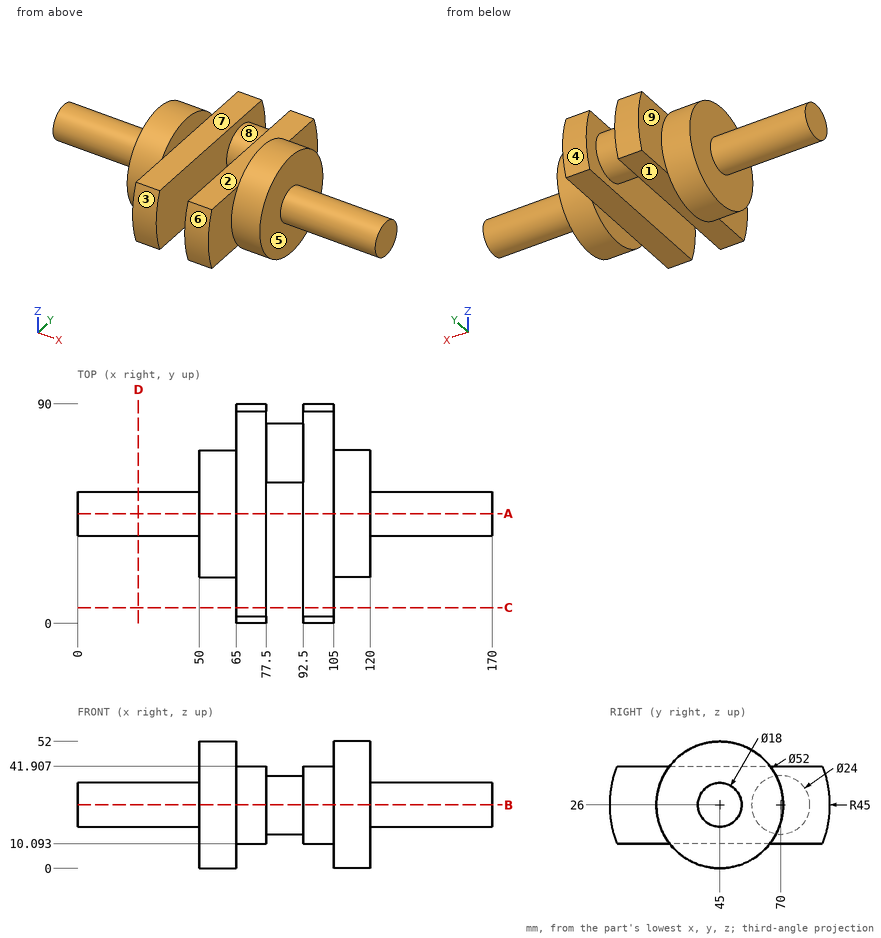
Check sheet for the drawn part. Datum: minimum x, y, z corner. Units: mm. A direction names the side the tool comes from. Give positions to 0.01 mm unless a question says otherwise; leave off trailing zeros. Loops run counter-clockwise (first coordinate to the right, second up) from the corner with the lowest first, then second, coordinate; pieces in that order, holes last.
1) Sectioned sample at D-D, the plane x = 25. Enter the section's corners in (y, z).
2) Thickness scan on line 1 along X through (y, z) = (28, 44); line 2 along X through (y, z) = (7.5, 17.5); line 3 along Z through (x, y) = (68.5, 73). Record the ranges inside material, lowest first.
3) Draft check along X on the marked faces 6, 7, 8 and 9. Enter one of: pulls with the +X half, pulls with the -X half, needs draft (parallel to the pull), parting line crosses it, or undercut.
4) Set-up check for the marked faces 1, 2, 3, 4 and 5: record each of +Z, -Z, +X, -X, +Y, -Y from which the full face is reachable in a straight line by a thin tool's end or side.
5) Sectioned sample at B-B, the plane z = 26. Enter the section's corners in (x, y), then the cut area to 3 significant figures.
6) Depth check by flat-ended pin: pin 1 Ø3 at (x, z) = (57.5, 29.5) entering from +Y; pin 2 Ø10 at (x, y) = (117.5, 16.5) entering from -Z (1 decimal); pin 3 Ø8 at (y, z) = (18.5, 45) entering from -X. Enter the tip coordinate at first touch or a pass-through.
7) Sectioned sample at A-A, the plane y = 45. Enter the section's corners in (x, z).
8) Sectioned sample at C-C, the plane y = 6.5. Enter the section's corners in (x, z), then the cut area to 3 significant figures.
Answers:
1. outline: circle Ø18 at (45, 26)
2. line 1: x = 50 to 65, 105 to 120
2. line 2: x = 65 to 77.5, 92.5 to 105
2. line 3: z = 10.09 to 41.91
3. face 6: needs draft
3. face 7: undercut
3. face 8: undercut
3. face 9: pulls with the -X half
4. face 1: -Z, +Y, -Y
4. face 2: +Z, +Y, -Y
4. face 3: +X, -X, -Y
4. face 4: +X, -X, +Y
4. face 5: +X
5. outline: (0, 36) - (50, 36) - (50, 19) - (65, 19) - (65, 0) - (77.5, 0) - (77.5, 58) - (92.5, 58) - (92.5, 0) - (105, 0) - (105, 19) - (120, 19) - (120, 36) - (170, 36) - (170, 54) - (120, 54) - (120, 71) - (105, 71) - (105, 90) - (92.5, 90) - (92.5, 82) - (77.5, 82) - (77.5, 90) - (65, 90) - (65, 71) - (50, 71) - (50, 54) - (0, 54) - close
5. area: 5,970 mm2
6. pin 1: stops at y = 70.92
6. pin 2: stops at z = 14.9
6. pin 3: stops at x = 65
7. outline: (0, 17) - (50, 17) - (50, 0) - (65, 0) - (65, 10.09) - (77.5, 10.09) - (77.5, 41.91) - (65, 41.91) - (65, 52) - (50, 52) - (50, 35) - (0, 35) - close; (92.5, 10.09) - (105, 10.09) - (105, 0) - (120, 0) - (120, 17) - (170, 17) - (170, 35) - (120, 35) - (120, 52) - (105, 52) - (105, 41.91) - (92.5, 41.91) - close
8. outline: (65, 10.09) - (77.5, 10.09) - (77.5, 41.91) - (65, 41.91) - close; (92.5, 10.09) - (105, 10.09) - (105, 41.91) - (92.5, 41.91) - close
8. area: 795 mm2
